The model under review builds one solid part; all positions refer to its coordinate system, in mm. A direction names the side the tool comes from. Give positions to 0.01 mm unless a question says otherwise; leave off trailing zeros. Loops run counter-clockwise (first coordinate to the right, second up) from the corner with the lowest first, then second, coordinate; pieces in that order, holes last. Notation, with made-up numbers: (-25.5, 32.25) -> (13.5, 32.25) arc R24 cw to (13.5, 55.25) -> close; hole circle Ø1 at (8, 84.5). An arc over 180 degrees is marked (long way). Write each question's results on one line, items separated by ' | '. Start each with the question number.
Q1. Mouldability with a two-part tool opening along X and no side actions: class faces 4 (the face through (-10.16, -12, 15)), 5 (the face through (-6, 15.231, 15)), 6 (the face through (12.7, -3, 15)) as released by +X, released by -X, zero draft, split by the parting line, or undercut.
Q2. We need section A-A (z = 7.62). Write out the cut boundary in (x, y), plus the area to 3 significant figures.
Q3. We need section D-D (x = -17). Write out the cut boundary in (y, z).
Q4. Insertion check: pin 1 Ø3 at (x, z) = (-8.5, 21.5) entering from -Y. The pin has a flat end and moves straight along its axis. Give the tip position at first contact, or say it passes through.
Q5. We need section C-C (y = -7). Write out the cut boundary in (x, z), plus the area to 3 significant figures.
Q6. Machinability: for faces 1 (the face through (0, -11, 15)), 2 (the face through (6.4, -11.8, 25.5)), 3 (the face through (-20.32, 0, 15)), which of the approach directions +Z, -Z, +X, -X, +Y, -Y give a long, thin tool a straight path to every point of the face, cutting with its end or side? Answer none if there is none.
Q7. Wall thickness on L1, parallel to Z at x = 8, y = -11.5; L2, parallel to X at y = -14, z = 11.5; L3, parallel to Y at x = -9.5, z = 9: over which ranges is each line inside the solid? List them lowest first. Write a range as [from, to].
Q8. We need section B-B (y = -11.43). Write out the cut boundary in (x, z), plus the area to 3 significant figures.
from build123d import *

# Parameters (mm, degrees)
F1_DEPTH = 30.48
F2_R     = 2.667
F3_DEPTH = 12.7
F4_R     = 5.08


with BuildPart() as f1:
    # F0 (on Top) → F1 (new body)
    with BuildSketch(Plane.XY):
        Polygon((-10.16, -16.51), (-10.16, -6.35), (0, -6.35), (0, -16.51), (12.7, -16.51), (12.7, -6.35), (12.7, 15.231052), (-17.145, 15.231052), (-20.32, 15.231052), (-20.32, -16.51), (-16.51, -16.51), align=None)
        with BuildLine():
            ThreePointArc((-13.462, 10.370257), (-14.354739, 8.214996), (-16.51, 7.322257))
            ThreePointArc((-16.51, 7.322257), (-18.665261, 12.525519), (-13.462, 10.370257))
        make_face(mode=Mode.SUBTRACT)
    extrude(amount=F1_DEPTH)

    # F2 (on face) → F3 (cut, through all)
    with BuildSketch(Plane.YZ.offset(12.7)):
        with Locations((-11.43, 22.86)):
            Circle(F2_R)
        with Locations((-11.43, 7.62)):
            Circle(F2_R)
    extrude(amount=-F3_DEPTH, mode=Mode.SUBTRACT)

    # F4
    f4_edges = [f1.edges().sort_by_distance(p)[0] for p in [
        (12.7, 15.231052, 15.24),
    ]]
    fillet(f4_edges, radius=F4_R)


solid = f1.part
Output:
1) face 4: undercut | face 5: zero draft | face 6: released by +X
2) outline: (-20.32, -16.51) -> (-10.16, -16.51) -> (-10.16, -6.35) -> (0, -6.35) -> (0, -8.76) -> (12.7, -8.76) -> (12.7, 10.15) arc R5.08 ccw to (7.62, 15.23) -> (-20.32, 15.23) -> close; (0, -16.51) -> (12.7, -16.51) -> (12.7, -14.1) -> (0, -14.1) -> close; hole (-16.51, 7.32) arc R3.05 ccw to (-13.46, 10.37) arc R3.05 ccw (long way) to start | area: 842 mm2
3) outline: (-16.51, 0) -> (7.36, 0) -> (7.36, 30.48) -> (-16.51, 30.48) -> close; (13.38, 0) -> (15.23, 0) -> (15.23, 30.48) -> (13.38, 30.48) -> close
4) pin 1: y = -6.35
5) outline: (-20.32, 0) -> (-10.16, 0) -> (-10.16, 30.48) -> (-20.32, 30.48) -> close; (0, 0) -> (12.7, 0) -> (12.7, 30.48) -> (0, 30.48) -> close | area: 697 mm2
6) face 1: +Z, -Z, -Y | face 2: +X | face 3: +Z, -Z, -X, +Y, -Y
7) L1: [0, 4.95], [10.29, 20.19], [25.53, 30.48] | L2: [-20.32, -10.16], [0, 12.7] | L3: [-6.35, 15.23]
8) outline: (-20.32, 0) -> (-10.16, 0) -> (-10.16, 30.48) -> (-20.32, 30.48) -> close; (0, 0) -> (12.7, 0) -> (12.7, 4.95) -> (0, 4.95) -> close; (0, 10.29) -> (12.7, 10.29) -> (12.7, 20.19) -> (0, 20.19) -> close; (0, 25.53) -> (12.7, 25.53) -> (12.7, 30.48) -> (0, 30.48) -> close | area: 561 mm2
